Read the model definition and answer for the solid it produces. Units are mm, in the model's axes. Face numbers are marked on the shaded views. A direction names the side the tool comes from. Coordinates: 2 decimals unless noted, no trailing zeros. Loops run counter-clockwise (first coordinate to the right, second up) from the corner with the lowest first, then second, coordinate; pieces in that order, holes last.
Q1. Flat-ended cylindrical pins translate along their axes: P1, Ø2, axis at x = -30.5, y = -0.5, coming from the +Z side; P2, Ø1.3, axis at x = 2.8, y = 0, coming from the +Z side; P3, Ø2, axis at x = 3, y = -0.5, coming from the -Z side; P4, Ø1.6, axis at y = 1, z = -15.5, coming from the +X side. Find the tip coordinate at first contact, or state that the pin passes through.
Q2. Section B-B (x = -20) is taken. Give the vertices of the cut face in (y, z), then the cut area to 3 significant figures.
Q3. Section A-A (z = -27) is taken. Give the vertices of the cut face in (x, y).
Q4. Section C-C (y = 0.65) is taken. Count the separate pieces of the cut face and the enclosed holes in it, then the cut area to 3 significant figures.
Q5. Straight lines are drawn through the part: line 1 (Z direction, x = 3.5, y = 1.75); line 2 (Y direction, x = 2.8, z = -27.5); line 3 (X direction, y = -0.1, z = -27). For each, find the intervals that lie inside material, in ascending order.
Q6. Which of the six approach directions +Z, -Z, +X, -X, +Y, -Y give full straight-line access (tool end or side, diameter ignored) to the marked faces 1 and 2?
Q7. Section D-D (z = -13.5) is taken. Give the vertices of the cut face in (x, y), then the cut area to 3 significant figures.
from build123d import *

# Parameters (mm, degrees)
SKETCH_1_R              = 1.1
EXTRUDE_1_DEPTH         = 2
EXTRUDE_2_DEPTH         = 8
EXTRUDE_START           = -22
EXTRUDE_3_DEPTH         = 8
HOLE_WIZARD_2_2_2_2_1_D = 2.2


with BuildPart() as part:
    # 草图1 → 凸台-拉伸1 (new body)
    with BuildSketch(Plane(origin=(0, 0, 0), x_dir=(1, 0, 0), z_dir=(0, 1, 0))):
        with BuildLine():
            Line((0, 30), (0, 0))
            Line((0, 0), (5, 0))
            Line((5, 0), (36.416208358, 23.812220652))
            ThreePointArc((36.416208358, 23.812220652), (37.768928241, 28.339843241), (33.861821998, 30.997612643))
            Line((33.861821998, 30.997612643), (5, 30))
            Line((5, 30), (0, 30))
        make_face()
        with BuildLine():
            Line((5, 6.273959963), (5, 24.997014021))
            Line((5, 24.997014021), (24.577554456, 25.673714745))
            ThreePointArc((24.577554456, 25.673714745), (26.531107578, 24.344830044), (25.854747636, 22.08101875))
            Line((25.854747636, 22.08101875), (5, 6.273959963))
        make_face(mode=Mode.SUBTRACT)
        with Locations(Location((34, 27, 0), (0, 0, 270))):
            Circle(SKETCH_1_R, mode=Mode.SUBTRACT)
    extrude(amount=EXTRUDE_1_DEPTH)

    # 圆角1
    # a fillet whose section is not a circle: 3 mm, written as the material it adds along each edge (its section moved 0.00015 mm through the faces so that the kernel can cut it)
    with BuildSketch(Plane(origin=(5, 0, -6.273959963), x_dir=(-2.4841613370279438e-05, 0, -0.999999999691447), z_dir=(0, 1, 0))) as fillet_1_piece_1:
        with BuildLine():
            add(Edge.make_bspline([(6.038255155, 0), (5.16698511, 2.1644e-05), (4.295715065, 4.3288e-05), (2.48642459, -0.523937582), (1.919396592, -1.665153012), (2.594631071, -3.423603004), (3.120906314, -4.117970242), (3.647181556, -4.81233748)], knots=[0, 0, 0, 0, 0, 0, 0.5, 0.5, 1, 1, 1, 1, 1, 1], degree=5))
            Line((3.647181556, -4.81233748), (3.599363965, -4.848579417))
            ThreePointArc((3.599363965, -4.848579417), (1.775832959, -2.442365375), (-0.047817591, -0.036241938))
            Line((-0.047817591, -0.036241938), (1.49e-06, 0.06))
            ThreePointArc((1.49e-06, 0.06), (3.019129066, 0.059925), (6.038256646, 0.06))
            Line((6.038256646, 0.06), (6.038255155, 0))
        make_face()
    extrude(amount=2)
    with BuildSketch(Plane(origin=(5, 0, -24.997014021), x_dir=(-5.1758116243326517e-05, 0, 0.9999999986605487), z_dir=(0, 1, 0))) as fillet_1_piece_2:
        with BuildLine():
            add(Edge.make_bspline([(2.8980962, 0), (2.407927047, -2.537e-05), (1.917757895, -5.074e-05), (0.835707431, 0.203366759), (0.1742891, 0.842251897), (-0.066497099, 1.916604675), (-0.083455103, 2.406480399), (-0.100413106, 2.896356123)], knots=[0, 0, 0, 0, 0, 0, 0.5, 0.5, 1, 1, 1, 1, 1, 1], degree=5))
            Line((-0.100413106, 2.896356123), (-0.160377189, 2.894280349))
            ThreePointArc((-0.160377189, 2.894280349), (-0.11009568, 1.446104883), (-0.059964082, -0.002075774))
            Line((-0.059964082, -0.002075774), (3.105e-06, -0.06))
            ThreePointArc((3.105e-06, -0.06), (1.449051202, -0.059925), (2.898099305, -0.06))
            Line((2.898099305, -0.06), (2.8980962, 0))
        make_face()
    extrude(amount=2)

    # 草图2 → 凸台-拉伸2 (add)
    with BuildSketch(Plane(origin=(0, 0, -30), x_dir=(-1, 0, 0), z_dir=(0, 0, -1))):
        with BuildLine():
            Line((0, 2), (2.8, 2))
            ThreePointArc((2.8, 2), (4.214213562, -1.414213562), (0.8, 0))
            Line((0.8, 0), (0, 0))
            Line((0, 0), (0, 2))
        make_face()
    extrude(amount=-EXTRUDE_2_DEPTH)

    # 草图2<2> → 凸台-拉伸3 (add)
    with BuildSketch(Plane(origin=(0, 0, -30), x_dir=(-1, 0, 0), z_dir=(0, 0, -1)).offset(EXTRUDE_START)):
        with BuildLine():
            Line((0, 2), (2.8, 2))
            ThreePointArc((2.8, 2), (4.214213562, -1.414213562), (0.8, 0))
            Line((0.8, 0), (0, 0))
            Line((0, 0), (0, 2))
        make_face()
    extrude(amount=-EXTRUDE_3_DEPTH)

    # Ø2.2 (2.2) 直径孔1 (through all)
    with Locations(Plane(origin=(0, 0, -30), x_dir=(-1, 0, 0), z_dir=(0, 0, -1))):
        with Locations((2.8, 0)):
            Hole(HOLE_WIZARD_2_2_2_2_1_D / 2)


with BuildPart() as body_2:
    # 镜向1: mirrored copy
    add(part.part.mirror(Plane(origin=(0, 0, 0), x_dir=(0, 0, 1), z_dir=(1, 0, 0))))


solid = body_2.part
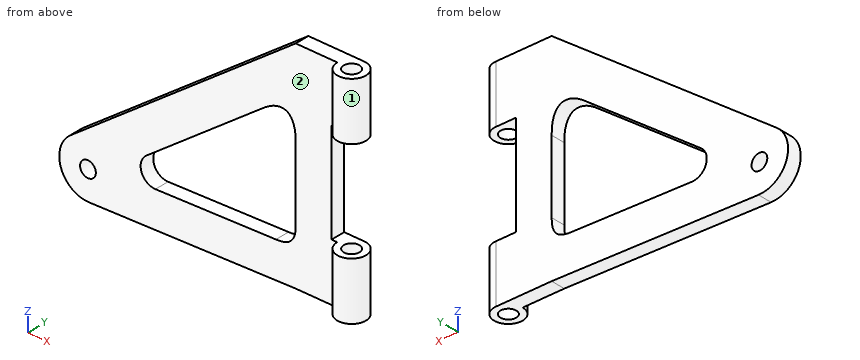
Numbers:
1. P1: stops at z = -18.67
1. P2: passes through
1. P3: stops at z = -30
1. P4: stops at x = 0
2. outline: (0, -30.52) - (2, -30.52) - (2, -25.52) - (0, -25.52) - close; (0, -17.64) - (2, -17.64) - (2, -11.37) - (0, -11.37) - close
2. area: 22.6 mm2
3. outline: (-38, 0) - (-35.1, 0) - (-35.1, 2) - (-38, 2) - close; (-32.9, 0) - (0.8, 0) arc R2 ccw (long way) to (2.8, 2) - (-32.9, 2) - close; hole circle Ø2.2 at (2.8, 0)
4. separate pieces: 3
4. enclosed holes: 2
4. area: 556 mm2
5. line 1: z = -30 to -22, -8 to 0
5. line 2: y = -2 to -1.1, 1.1 to 2
5. line 3: x = 0.8 to 1.7, 3.9 to 4.8
6. face 1: +Z, -Z
6. face 2: +Z, -Z, -X, -Y
7. outline: (-22.81, 0) - (-14.53, 0) - (-14.53, 2) - (-22.81, 2) - close; (-5, 0) - (0, 0) - (0, 2) - (-5, 2) - close
7. area: 26.6 mm2
